Answer from the drawing. Dimensions are ordinates in mm from the lowest x, y and z of the part. A direction names the side the tool comes from. Round coordinates to 2 decimals unless told otherwise and drop trailing zeros. Write each loop counter-clockwise with the first axis right and the second up, starting at its lowest first coordinate (ties: lowest second). Pieces come first, ordered by that corner, then holes. Notation, with made-up numbers: M -0.5,6.25 L 37.5,6.25 A12 ccw 37.5,11.25 Z; hole C 49.25,32.25 d3. An arc over 180 degrees is marked long. Answer as CSV lines item,"result". Start each with the question number.
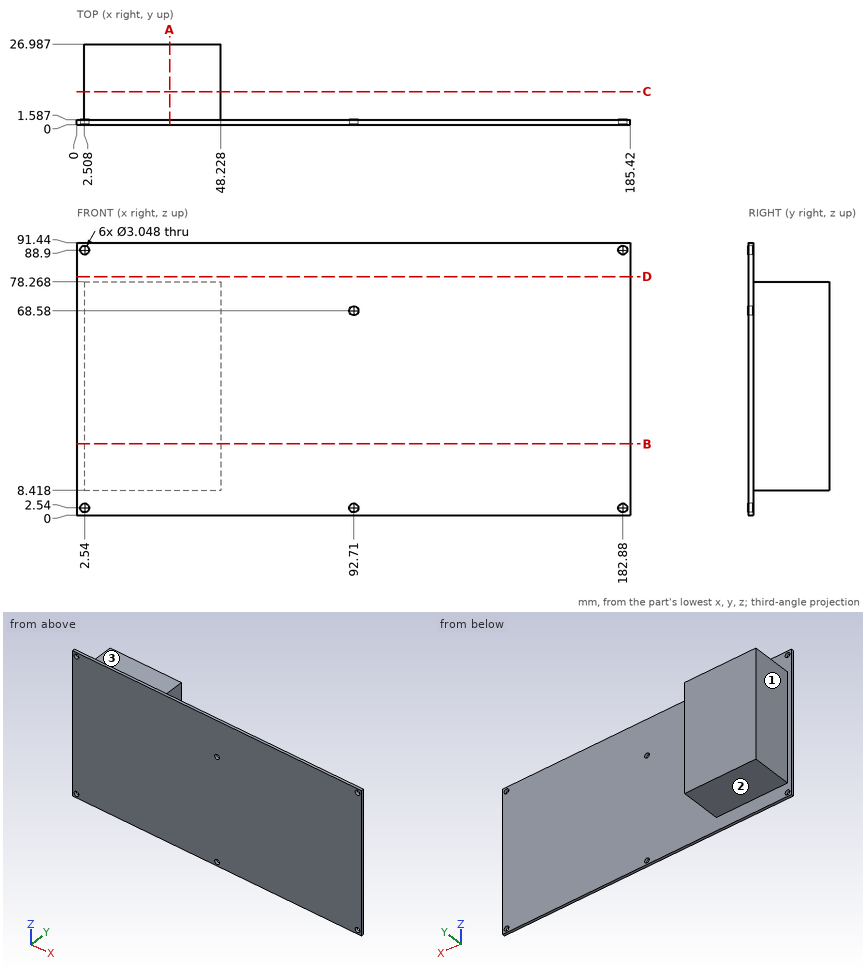
Q1. Find section B-B (z = 24). Determine the outline of the cut face in (x, y), plus the area to 3 significant figures.
Q2. Straight lines are drawn through the part: L1, parallel to X at y = 0.5, z = 88.9 (1 decimal); L2, parallel to Z at x = 92.71, y = 1.1 (1 decimal); L3, parallel to Z at x = 2.54, y = 1.15 (1 decimal). For each, find the intervals that lie inside material, in ascending order.
Q3. For the marked faces 1, 2 and 3, determine the directions among +Z, -Z, +X, -X, +Y, -Y from which every point of the face is accessible in a straight line to the end or side of a thin tool.
Q4. Each of these flat-tipped pins is pushed along its axis until it touches: P1, Ø5, axis at x = 2.54, z = 88.9, coming from the +Y side; P2, Ø7.5, axis at y = 16.5, z = 35.5, coming from the -X side; P3, Ø6, axis at y = 17, z = 46.5, coming from the +X side; P4, Ø2.5, axis at x = 92.71, z = 68.58, coming from the -Y side. Where does it stop, or does it pass through?
Q5. Find section D-D (z = 80). Determine the outline of the cut face in (x, y).
Q6. Find section A-A (x = 31). Determine the outline of the cut face in (y, z).
Q7. Find section C-C (y = 11). Determine the outline of the cut face in (x, z).
Reported:
1,outline,"M 0,0 L 185.42,0 L 185.42,1.59 L 48.23,1.59 L 48.23,26.99 L 2.51,26.99 L 2.51,1.59 L 0,1.59 Z"
1,area,"1,460 mm2"
2,L1,"x = 0 to 1, 4.1 to 181.4, 184.4 to 185.4"
2,L2,"z = 0 to 1, 4.1 to 67.1, 70.1 to 91.4"
2,L3,"z = 0 to 1, 4.1 to 87.4, 90.4 to 91.4"
3,face 1,"+Z, -Z, -X, +Y"
3,face 2,"-Z, +X, -X, +Y"
3,face 3,"+Z, +X, -X, +Y"
4,P1,"stops at y = 1.59"
4,P2,"stops at x = 2.51"
4,P3,"stops at x = 48.23"
4,P4,"passes through"
5,outline,"M 0,0 L 185.42,0 L 185.42,1.59 L 0,1.59 Z"
6,outline,"M 0,0 L 1.59,0 L 1.59,8.42 L 26.99,8.42 L 26.99,78.27 L 1.59,78.27 L 1.59,91.44 L 0,91.44 Z"
7,outline,"M 2.51,8.42 L 48.23,8.42 L 48.23,78.27 L 2.51,78.27 Z"
